Source: CAD feature listing. Evaluate the final solid. Frame: model axes, mm. Face numbers are marked on the shaded views. A direction names the side the tool comes from. Give positions to 0.01 mm unless a question says otherwise; leave off trailing zeros. Order: outer loops, then holes, each group sorted by start corner. A loop starts at its lowest first (then second) coordinate and runs counter-clockwise, first axis right, second up. Notation, with made-up numbers: (4.25, -1.5) - (51.25, -1.5) arc R14 ccw to (51.25, 14.5) - close; hole circle Ø6 at (-1, -36.75). An arc over 180 degrees is marked (long way). Write each question's results on one line, items separated by ' | '. Start each with the question number.
Item 1: Set-up query: the marked faces 1 and 2. Return all of +Z, -Z, +X, -X, +Y, -Y with unobstructed straight access to the full face (end or side cutting, diameter ignored); none if empty.
Item 2: Mould query, pull axis Y, two halves, no side actions, for the marked faces 3, 4, 5 and 6. Classes: released by +Y, released by -Y, zero draft, split by the parting line, or undercut.
Item 3: Section B-B on y = 0. Output: boundary loops of the cut face in (x, z).
Item 4: Line query: line 1 along X through (y, z) = (2, 15.5); line 2 along Y through (x, z) = (-13.5, 12); line 3 along X through (y, z) = (6.5, 18). Output: solid intervals per line, ascending.
Item 5: Section A-A on z = 8. Output: boundary loops of the cut face in (x, y).
Item 6: Section C-C on x = -13.5. Output: boundary loops of the cut face in (y, z), and give its area (3 significant figures).
Item 7: Contact query for a flat-ended pin moving along its axis: pin 1 Ø6.5 at (x, y) = (16, 1.5) entering from +Z. Output: stop coordinate, or through.
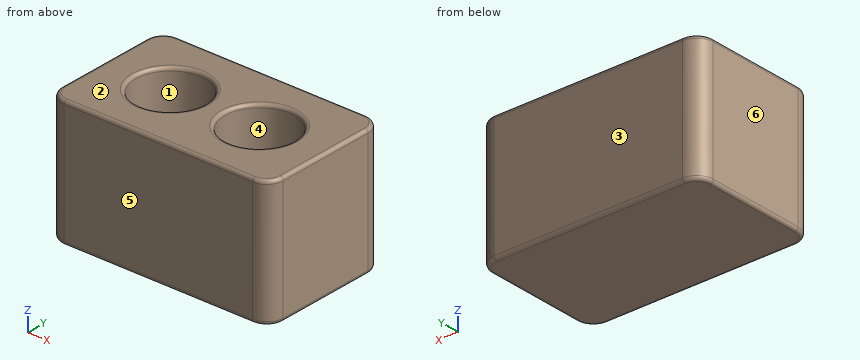
```python
from build123d import *

# Parameters (mm, degrees)
F0_W         = 67
F0_H         = 40
F0_R         = 10.5
F1_DEPTH     = 36
F2_W         = 67
F2_H         = 40
F3_DEPTH     = 2
F4_R         = 1
F5_T1_DEPTH  = 38
F5_T4_ANGLE  = 90
F5_T6_ANGLE  = 90
F5_T8_ANGLE  = 90
F5_T10_ANGLE = 90
F5_T12_ANGLE = 90
F5_T14_ANGLE = 90
F5_T16_ANGLE = 90
F5_T18_ANGLE = 90


# Not quite as in the source:
# - a fillet or chamfer that OpenCascade refuses, or shapes differently, is made with other operations: its cross-section is extruded or revolved along the edge and cut away or added


with BuildPart() as f1:
    # F0 (on Top) → F1 (new body)
    with BuildSketch(Plane.XY):
        Rectangle(F0_W, F0_H)
        with Locations((-13.5, 0)):
            Circle(F0_R, mode=Mode.SUBTRACT)
        with Locations((13.5, 0)):
            Circle(F0_R, mode=Mode.SUBTRACT)
    extrude(amount=F1_DEPTH)

    # F2 (on face) → F3 (join)
    with BuildSketch(Plane(origin=(0, 0, 0), x_dir=(1, 0, 0), z_dir=(0, 0, -1))):
        Rectangle(F2_W, F2_H)
    extrude(amount=F3_DEPTH)

    # F4
    f4_edges = [f1.edges().sort_by_distance(p)[0] for p in [
        (0, 20, 36),
        (-33.5, 0, 36),
        (0, -20, 36),
        (33.5, 0, 36),
        (-24, 0, 36),
        (3, 0, 36),
        (0, 20, -2),
        (33.5, 0, -2),
        (0, -20, -2),
        (-33.5, 0, -2),
    ]]
    fillet(f4_edges, radius=F4_R)

    # F5: fillet of radius 5 on 4 edges, made by hand

    # F5_s2 → F5_t1 (cut)
    with BuildSketch(Plane.XY.offset(-2)):
        with BuildLine():
            ThreePointArc((28.5, 20), (32.0355339059, 18.5355339059), (33.5, 15))
            Line((33.5, 15), (33.5, 20))
            Line((33.5, 20), (28.5, 20))
        make_face()
        with BuildLine():
            ThreePointArc((33.5, -15), (32.0355339059, -18.5355339059), (28.5, -20))
            Line((28.5, -20), (33.5, -20))
            Line((33.5, -20), (33.5, -15))
        make_face()
        with BuildLine():
            ThreePointArc((-33.5, -15), (-32.0355339059, -18.5355339059), (-28.5, -20))
            Line((-28.5, -20), (-33.5, -20))
            Line((-33.5, -20), (-33.5, -15))
        make_face()
        with BuildLine():
            ThreePointArc((-28.5, 20), (-32.0355339059, 18.5355339059), (-33.5, 15))
            Line((-33.5, 15), (-33.5, 20))
            Line((-33.5, 20), (-28.5, 20))
        make_face()
    extrude(amount=F5_T1_DEPTH, mode=Mode.SUBTRACT)

    # F5_s3 → F5_t4 (revolve, cut)
    with BuildSketch(Plane.XZ.offset(-15)):
        with BuildLine():
            ThreePointArc((-32.5, -2), (-33.2071067812, -1.7071067812), (-33.5, -1))
            Line((-33.5, -1), (-33.5, -2))
            Line((-33.5, -2), (-32.5, -2))
        make_face()
    revolve(axis=Axis((-28.5, 15, -2), (0, 0, -1)), revolution_arc=F5_T4_ANGLE, mode=Mode.SUBTRACT)

    # F5_s5 → F5_t6 (revolve, cut)
    with BuildSketch(Plane.YZ.offset(-28.5)):
        with BuildLine():
            ThreePointArc((19, 36), (19.7071067812, 35.7071067812), (20, 35))
            Line((20, 35), (20, 36))
            Line((20, 36), (19, 36))
        make_face()
    revolve(axis=Axis((-28.5, 15, 36), (0, 0, 1)), revolution_arc=F5_T6_ANGLE, mode=Mode.SUBTRACT)

    # F5_s7 → F5_t8 (revolve, cut)
    with BuildSketch(Plane.YZ.offset(-28.5)):
        with BuildLine():
            ThreePointArc((-19, -2), (-19.7071067812, -1.7071067812), (-20, -1))
            Line((-20, -1), (-20, -2))
            Line((-20, -2), (-19, -2))
        make_face()
    revolve(axis=Axis((-28.5, -15, -2), (0, 0, -1)), revolution_arc=F5_T8_ANGLE, mode=Mode.SUBTRACT)

    # F5_s9 → F5_t10 (revolve, cut)
    with BuildSketch(Plane.XZ.offset(15)):
        with BuildLine():
            ThreePointArc((-32.5, 36), (-33.2071067812, 35.7071067812), (-33.5, 35))
            Line((-33.5, 35), (-33.5, 36))
            Line((-33.5, 36), (-32.5, 36))
        make_face()
    revolve(axis=Axis((-28.5, -15, 36), (0, 0, 1)), revolution_arc=F5_T10_ANGLE, mode=Mode.SUBTRACT)

    # F5_s11 → F5_t12 (revolve, cut)
    with BuildSketch(Plane.YZ.offset(28.5)):
        with BuildLine():
            ThreePointArc((-19, 36), (-19.7071067812, 35.7071067812), (-20, 35))
            Line((-20, 35), (-20, 36))
            Line((-20, 36), (-19, 36))
        make_face()
    revolve(axis=Axis((28.5, -15, 36), (0, 0, 1)), revolution_arc=F5_T12_ANGLE, mode=Mode.SUBTRACT)

    # F5_s13 → F5_t14 (revolve, cut)
    with BuildSketch(Plane.XZ.offset(15)):
        with BuildLine():
            ThreePointArc((32.5, -2), (33.2071067812, -1.7071067812), (33.5, -1))
            Line((33.5, -1), (33.5, -2))
            Line((33.5, -2), (32.5, -2))
        make_face()
    revolve(axis=Axis((28.5, -15, -2), (0, 0, -1)), revolution_arc=F5_T14_ANGLE, mode=Mode.SUBTRACT)

    # F5_s15 → F5_t16 (revolve, cut)
    with BuildSketch(Plane.XZ.offset(-15)):
        with BuildLine():
            ThreePointArc((32.5, 36), (33.2071067812, 35.7071067812), (33.5, 35))
            Line((33.5, 35), (33.5, 36))
            Line((33.5, 36), (32.5, 36))
        make_face()
    revolve(axis=Axis((28.5, 15, 36), (0, 0, 1)), revolution_arc=F5_T16_ANGLE, mode=Mode.SUBTRACT)

    # F5_s17 → F5_t18 (revolve, cut)
    with BuildSketch(Plane.YZ.offset(28.5)):
        with BuildLine():
            ThreePointArc((19, -2), (19.7071067812, -1.7071067812), (20, -1))
            Line((20, -1), (20, -2))
            Line((20, -2), (19, -2))
        make_face()
    revolve(axis=Axis((28.5, 15, -2), (0, 0, -1)), revolution_arc=F5_T18_ANGLE, mode=Mode.SUBTRACT)


solid = f1.part
```
Evaluation:
1) face 1: +Z | face 2: +Z, +X, -X, +Y, -Y
2) face 3: released by +Y | face 4: undercut | face 5: released by -Y | face 6: zero draft
3) outline: (-33.5, -1) arc R1 ccw to (-32.5, -2) - (32.5, -2) arc R1 ccw to (33.5, -1) - (33.5, 35) arc R1 ccw to (32.5, 36) - (25, 36) arc R1 ccw to (24, 35) - (24, 0) - (3, 0) - (3, 35) arc R1 ccw to (2, 36) - (-2, 36) arc R1 ccw to (-3, 35) - (-3, 0) - (-24, 0) - (-24, 35) arc R1 ccw to (-25, 36) - (-32.5, 36) arc R1 ccw to (-33.5, 35) - close
4) line 1: x = -33.5 to -23.81, -3.19 to 3.19, 23.81 to 33.5 | line 2: y = -20 to -10.5, 10.5 to 20 | line 3: x = -33.5 to -21.75, -5.25 to 5.25, 21.75 to 33.5
5) outline: (-33.5, -15) arc R5 ccw to (-28.5, -20) - (28.5, -20) arc R5 ccw to (33.5, -15) - (33.5, 15) arc R5 ccw to (28.5, 20) - (-28.5, 20) arc R5 ccw to (-33.5, 15) - close; hole circle Ø21 at (-13.5, 0); hole circle Ø21 at (13.5, 0)
6) outline: (-20, -1) arc R1 ccw to (-19, -2) - (19, -2) arc R1 ccw to (20, -1) - (20, 35) arc R1 ccw to (19, 36) - (11.5, 36) arc R1 ccw to (10.5, 35) - (10.5, 0) - (-10.5, 0) - (-10.5, 35) arc R1 ccw to (-11.5, 36) - (-19, 36) arc R1 ccw to (-20, 35) - close | area: 763 mm^2
7) pin 1: stops at z = 0
